Source: CAD feature listing. Evaluate the final solid. Frame: model axes, mm. Face numbers are marked on the shaded views. A direction names the side the tool comes from. Round coordinates to 2 decimals unless told otherwise and drop trailing zeros. Write each loop counter-clockwise with the first axis right and the second up, starting at its lowest first coordinate (ties: lowest second). Pieces come first, ordered by that corner, then holes. Notation, with made-up numbers: M 54.5,-15 L 73.5,-15 A12 ccw 73.5,-1 Z; hole C -34,55 d2. An arc over 180 degrees is marked long. Answer in a Markdown table with one row per item. Add a question column.
Item 1: Contact query for flat-ended pins moving along their axis: pin 1 (1.5 mm diameter, centred on y = -24, z = 24, fed in from -X); pin 2 (5 mm diameter, centred on y = -28, z = 4.5, fed in from -X); pin 3 (5 mm diameter, centred on x = 63.5, y = -19, fed in from +Z). Output: stop coordinate, or through.
Item 2: Mould query, pull axis X, two halves, no side actions, for the marked faces 1, 2 and 3. Classes: released by +X, released by -X, zero draft, split by the parting line, or undercut.
Item 3: Set-up query: the marked faces 4, 5 and 6. Return all of +Z, -Z, +X, -X, +Y, -Y with unobstructed straight access to the full face (end or side cutting, diameter ignored); none if empty.
Item 4: Material intervals for probe 1 along X at (y, z) = (-29, 16.5); probe 2 along Y at (x, z) = (56, 7.5); probe 3 along Z at (x, y) = (61, -8), sorted ascending.
Item 5: Cut plane D-D on x = 23. Return loops of the section in (y, z), and give its area (3 significant figures).
Item 6: Cut plane A-A on x = 65. Return loops of the section in (y, z), and give its area (3 significant figures).
Item 7: Cut plane C-C on z = 25. Return loops of the section in (x, y).
Item 8: Cut plane B-B on y = -33.5. Return loops of the section in (x, z), and give its area (3 significant figures).
from build123d import *

# Parameters (mm, degrees)
F1_DEPTH = 30
F3_DEPTH = 10
F5_DEPTH = 43.3


with BuildPart() as f1:
    # F0 (on Front) → F1 (new body)
    with BuildSketch(Plane.XZ):
        Polygon((10, 10), (0, 0), (80, 0), (70, 10), (60, 10), (60, 40), (20, 40), (20, 10), align=None)
    extrude(amount=F1_DEPTH)

    # F2 (on face) → F3 (join)
    with BuildSketch(Plane.XZ.offset(30)):
        with BuildLine():
            Line((60, 40), (20, 40))
            ThreePointArc((20, 40), (40, 20), (60, 40))
        make_face()
    extrude(amount=F3_DEPTH)

    # F4 (on face) → F5 (cut)
    with BuildSketch(Plane.XZ.offset(40)):
        with BuildLine():
            ThreePointArc((30, 40), (40, 30), (50, 40))
            Line((50, 40), (30, 40))
        make_face()
    extrude(amount=-F5_DEPTH, mode=Mode.SUBTRACT)


solid = f1.part
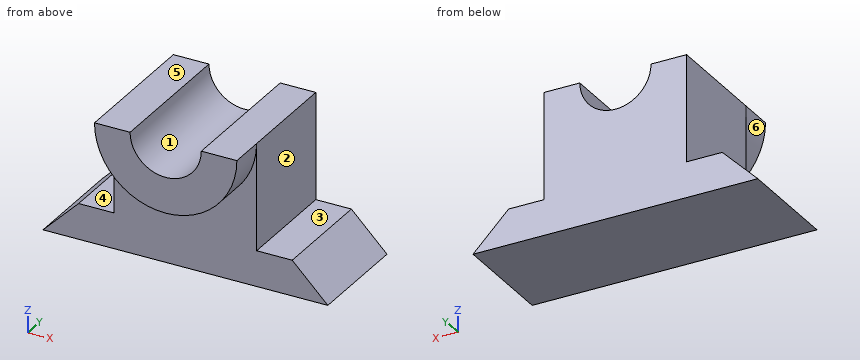
Results below:
| question | item | result |
|---|---|---|
| 1 | pin 1 | x = 20 |
| 1 | pin 2 | x = 2 |
| 1 | pin 3 | z = 10 |
| 2 | face 1 | undercut |
| 2 | face 2 | released by +X |
| 2 | face 3 | zero draft |
| 3 | face 4 | +Z, -X, +Y, -Y |
| 3 | face 5 | +Z, +X, -X, +Y, -Y |
| 3 | face 6 | -Z, -Y |
| 4 | probe 1 | 20 to 60 |
| 4 | probe 2 | -30 to 0 |
| 4 | probe 3 | 0 to 10 |
| 5 | outline | M -40,29.46 L -30,29.46 L -30,0 L 0,0 L 0,40 L -40,40 Z |
| 5 | area | 1,310 mm2 |
| 6 | outline | M -30,0 L 0,0 L 0,10 L -30,10 Z |
| 6 | area | 300 mm2 |
| 7 | outline | M 20,-30 L 26.77,-30 L 26.77,-40 L 53.23,-40 L 53.23,-30 L 60,-30 L 60,0 L 20,0 Z |
| 8 | outline | M 20,40 A20 ccw 60,40 L 50,40 A10 cw 30,40 Z |
| 8 | area | 471 mm2 |
